Part model, mm, in its own coordinate system. A direction names the side the tool comes from. Round coordinates to 2 decimals unless told otherwise and drop trailing zeros. Write each loop counter-clockwise with the first axis right and the second up, starting at its lowest first coordinate (ties: lowest second). Pieces come first, ordered by that corner, then holes. Notation, with made-up numbers: M -15.75,52 L 10.25,52 A32 cw 10.25,83 Z; hole C -11.75,74.25 d7. An arc over 180 degrees is marked long. Answer as a JSON object with one key per item and string values. Group by question number.
1. Band-saw the part on A-A, the plane z = -33.5. Write the cut outline in (x, y).
2. Drop flat-ended pins along their axis: pin 1 (2.5 mm diameter, centred on x = 39, z = -44, fed in from -Y); pin 2 (4 mm diameter, centred on x = 16.5, y = -14.5, fed in from -Z); pin 3 (3.5 mm diameter, centred on x = 38, z = -44, fed in from +Y). Give the stop position or say it passes through.
3. Band-saw the part on C-C, the plane x = 32. Write the cut outline in (y, z).
4. Two-plate mould, pull along X, no slides. Class faces 4 (the face through (20, -7, -38.658)), 5 (the face through (39, 4.716, -44)), 6 (the face through (0.6, -39.71, -12.03)), 7 (the face through (38.5, -9, -12)): +X half, -X half, draft (parallel to the pull), parting line (faces both ways), or undercut.
5. Band-saw the part on B-B, the plane y = -13.5. Write the cut outline in (x, z), plus the area to 3 significant figures.
6. Band-saw the part on D-D, the plane y = -31.5. Write the cut outline in (x, z).
7. Drill centre lines: line 1 (Y direction, x = 7, z = -18.5); line 2 (X direction, y = 6, z = -21.5); line 3 (X direction, y = -34.5, z = -25.5). Where is each one in solid material? Low to high. Write a range as from..to.
8. Which spindle directions (+Z, -Z, +X, -X, +Y, -Y) get a long thin tool onto all of the face, cutting with end or side? Do faces 1 (the face through (-0.986, -23.342, -2.205)), 2 (the face through (-0.986, -24.964, -21.046)), 3 (the face through (37, -7, 20)). Say none if no direction does.
from build123d import *

# Parameters (mm, degrees)
SKETCH1_W           = 55
SKETCH1_H           = 65
BOSS_EXTRUDE1_DEPTH = 40
SKETCH2_W           = 37
SKETCH2_H           = 62
CUT_EXTRUDE1_DEPTH  = 53.5
FILLET1_R           = 2
FILLET7_R           = 2
BOSS_EXTRUDE2_DEPTH = 2
SKETCH17_R          = 0.75
CUT_EXTRUDE3_DEPTH  = 3.5
SKETCH18_W          = 3
SKETCH18_H          = 25
BOSS_EXTRUDE3_DEPTH = 7
SKETCH19_W          = 3
SKETCH19_H          = 25
BOSS_EXTRUDE4_DEPTH = 7
SKETCH22_W          = 3
SKETCH22_H          = 25
BOSS_EXTRUDE5_DEPTH = 1.5
SKETCH23_W          = 3
SKETCH23_H          = 21
CUT_EXTRUDE4_DEPTH  = 3
FILLET9_R           = 10
SKETCH24_W          = 3
SKETCH24_H          = 20
CUT_EXTRUDE5_DEPTH  = 5


with BuildPart() as part:
    # Sketch1 → Boss-Extrude1 (new body)
    with BuildSketch(Plane(origin=(0, 0, 0), x_dir=(0, 0, -1), z_dir=(1, 0, 0))):
        with Locations((12.658301158, -7.783783784)):
            Rectangle(SKETCH1_W, SKETCH1_H)
    extrude(amount=BOSS_EXTRUDE1_DEPTH)

    # Sketch2 → Cut-Extrude1 (cut)
    with BuildSketch(Plane.XY.offset(14.841698842)):
        with Locations((20, -7.783783784)):
            Rectangle(SKETCH2_W, SKETCH2_H)
    extrude(amount=-CUT_EXTRUDE1_DEPTH, mode=Mode.SUBTRACT)

    # Fillet1
    fillet1_edges = [part.edges().sort_by_distance(p)[0] for p in [
        (40, 24.716216216, -12.658301158),
        (0, -7.783783784, -40.158301158),
        (0, -40.283783784, -12.658301158),
        (20, 24.716216216, -40.158301158),
        (20, -40.283783784, -40.158301158),
        (40, -40.283783784, -12.658301158),
    ]]
    fillet(fillet1_edges, radius=FILLET1_R)

    # Fillet7
    # the kernel refuses this fillet: 2 mm, written as the material it takes off along each edge
    with BuildSketch(Plane(origin=(2, 22.716216216, -38.158301158), x_dir=(-1, 0, 0), z_dir=(0, 1, 0))) as fillet7_piece_1_section:
        Polygon((0, 0), (FILLET7_R, 0), (FILLET7_R, -FILLET7_R), (0, -FILLET7_R), align=None)
    fillet7_piece_1 = extrude(amount=FILLET7_R, mode=Mode.PRIVATE)
    fillet7_piece_1 = fillet7_piece_1 - Plane(origin=(2, 22.716216216, -38.158301158), x_dir=(0.7071067811865475, 0, 0.7071067811865475), z_dir=(0, 1, 0)) * Sphere(FILLET7_R, mode=Mode.PRIVATE)
    add(fillet7_piece_1, mode=Mode.SUBTRACT)
    with BuildSketch(Plane(origin=(0, 24.716216216, 19.841698842), x_dir=(1, 0, 0), z_dir=(0, 0, -1))) as fillet7_piece_2:
        with BuildLine():
            CenterArc((FILLET7_R, FILLET7_R), FILLET7_R, 180, 90)
            Line((0, FILLET7_R), (0, 0))
            Line((0, 0), (FILLET7_R, 0))
        make_face()
    extrude(amount=58, mode=Mode.SUBTRACT)

    # Sketch16 → Boss-Extrude2 (add)
    with BuildSketch(Plane.ZY):
        with BuildLine():
            ThreePointArc((-5.736624698, 17.653603477), (-12.555029292, 21.251157673), (-19.459260578, 17.82119736))
            ThreePointArc((-19.459260578, 17.82119736), (-22.577953623, 10.406366019), (-24.332801521, 2.556112585))
            ThreePointArc((-24.332801521, 2.556112585), (-24.205542572, -2.611001185), (-22.077609894, -7.321326234))
            ThreePointArc((-22.077609894, -7.321326234), (-19.565557127, -13.10020976), (-20.565766521, -19.321583006))
            ThreePointArc((-20.565766521, -19.321583006), (-21.037839736, -25.044648424), (-19.459260578, -30.565918092))
            ThreePointArc((-19.459260578, -30.565918092), (-10.406141283, -35.070804577), (-2.644818813, -28.588918684))
            ThreePointArc((-2.644818813, -28.588918684), (-2.212041027, -23.266864026), (-3.652018787, -18.125071882))
            ThreePointArc((-3.652018787, -18.125071882), (-4.916354141, -12.558379885), (-2.644818813, -7.321326234))
            ThreePointArc((-2.644818813, -7.321326234), (-1.085145754, -3.293973241), (-0.88318994, 1.020116006))
            ThreePointArc((-0.88318994, 1.020116006), (-2.121330664, 9.683670911), (-5.736624698, 17.653603477))
        make_face()
    extrude(amount=BOSS_EXTRUDE2_DEPTH)

    # Sketch17 → Cut-Extrude3 (cut)
    with BuildSketch(Plane.ZY.offset(2)):
        with Locations((-15.44953453, 14.297400207)):
            Circle(SKETCH17_R)
        with Locations((-13.44953453, 14.297400207)):
            Circle(SKETCH17_R)
        with Locations((-4.229257303, 6.228419053)):
            Circle(SKETCH17_R)
        with Locations((-6.229257303, 6.228419053)):
            Circle(SKETCH17_R)
        with Locations((-20.261021777, -0.629536007)):
            Circle(SKETCH17_R)
        with Locations((-18.261021777, -0.629536007)):
            Circle(SKETCH17_R)
        with Locations((-12.530672595, -28.291294223)):
            Circle(SKETCH17_R)
        with Locations((-10.530672595, -28.291294223)):
            Circle(SKETCH17_R)
    extrude(amount=-CUT_EXTRUDE3_DEPTH, mode=Mode.SUBTRACT)

    # Sketch18 → Boss-Extrude3 (add)
    with BuildSketch(Plane(origin=(0, 0, -40.158301158), x_dir=(-1, 0, 0), z_dir=(0, 0, -1))):
        with Locations((-38.5, -7.783783784)):
            Rectangle(SKETCH18_W, SKETCH18_H)
    extrude(amount=BOSS_EXTRUDE3_DEPTH)

    # Sketch19 → Boss-Extrude4 (add)
    with BuildSketch(Plane.XY.offset(14.841698842)):
        with Locations((38.5, -6.783783784)):
            Rectangle(SKETCH19_W, SKETCH19_H)
    extrude(amount=BOSS_EXTRUDE4_DEPTH)

    # Sketch22 → Boss-Extrude5 (add)
    with BuildSketch(Plane.ZY.offset(-38.5)):
        with Locations((13.341698842, -6.783783784)):
            Rectangle(SKETCH22_W, SKETCH22_H)
    extrude(amount=BOSS_EXTRUDE5_DEPTH)

    # Sketch23 → Cut-Extrude4 (cut)
    with BuildSketch(Plane.ZY.offset(-37)):
        with Locations((-43.658301158, -7.783783784)):
            Rectangle(SKETCH23_W, SKETCH23_H)
        with Locations((18.341698842, -6.783783784)):
            Rectangle(SKETCH23_W, SKETCH23_H)
    extrude(amount=-CUT_EXTRUDE4_DEPTH, mode=Mode.SUBTRACT)

    # Fillet9
    # the kernel refuses this fillet: 10 mm, written as the material it takes off along each edge
    with BuildSketch(Plane(origin=(37, 18.885783407, 11.841698842), x_dir=(0, 0, 1), z_dir=(0, -1, 0))) as fillet9_piece_1:
        with BuildLine():
            CenterArc((5.267826876, -10), FILLET9_R, 90, 31.788330617)
            Line((0, -1.5), (-0.105356538, -1.33))
            ThreePointArc((-0.105356538, -1.33), (-0.2, -0.75), (-0.2, 0))
            Line((-0.2, 0), (0, 0.2))
            Line((0, 0.2), (5.267826876, 0.2))
            Line((5.267826876, 0.2), (5.267826876, 0))
        make_face()
    extrude(amount=51.339134382, mode=Mode.SUBTRACT)

    # Sketch24 → Cut-Extrude5 (cut)
    with BuildSketch(Plane.XZ.offset(40.283783784)):
        with Locations((37, -12.658301158)):
            Rectangle(SKETCH24_W, SKETCH24_H)
    extrude(amount=-CUT_EXTRUDE5_DEPTH, mode=Mode.SUBTRACT)


solid = part.part
Worked answers:
{
 "1": {"outline": "M 0,-38.28 A2 ccw 2,-40.28 L 38,-40.28 A2 ccw 40,-38.28 L 40,22.72 A2 ccw 38,24.72 L 2,24.72 A2 ccw 0,22.72 Z; hole M 1.5,-38.78 L 38.5,-38.78 L 38.5,23.22 L 1.5,23.22 Z"},
 "2": {"pin 1": "stops at y = -20.28", "pin 2": "stops at z = -40.16", "pin 3": "stops at y = 4.72"},
 "3": {"outline": "M -40.28,-38.16 A2 ccw -38.28,-40.16 L 22.72,-40.16 A2 ccw 24.72,-38.16 L 24.72,14.84 L 23.22,14.84 L 23.22,-38.66 L -38.78,-38.66 L -38.78,14.84 L -40.28,14.84 Z"},
 "4": {"face 4": "undercut", "face 5": "draft", "face 6": "-X half", "face 7": "undercut"},
 "5": {"outline": "M -2,-19.52 L 0,-19.52 L 0,-38.16 A2 ccw 2,-40.16 L 37,-40.16 L 37,-42.16 L 40,-42.16 L 40,16.84 L 37,16.84 A10 ccw 38.5,11.84 L 38.5,-38.66 L 1.5,-38.66 L 1.5,14.84 L 0,14.84 L 0,-4.96 L -2,-4.96 Z; M 37,-47.16 L 40,-47.16 L 40,-45.16 L 37,-45.16 Z; M 37,19.84 L 40,19.84 L 40,21.84 L 37,21.84 Z", "area": "275 mm^2"},
 "6": {"outline": "M -2,-18.83 L 0,-18.83 L 0,-38.16 A2 ccw 2,-40.16 L 40,-40.16 L 40,14.84 L 38.5,14.84 L 38.5,-38.66 L 1.5,-38.66 L 1.5,14.84 L 0,14.84 L 0,-4.14 L -2,-4.14 Z"},
 "7": {"line 1": "y = -40.28..-38.78, 23.22..24.72", "line 2": "x = -2..1.5, 38.5..40", "line 3": "x = 0..1.5, 38.5..40"},
 "8": {"face 1": "+Z, -X", "face 2": "-Z, -X", "face 3": "+Z, -X, +Y, -Y"}
}
